Geometry: see drawing. Coordinates: mm, zero at the bounding-box minimum. A direction names the side the tool comes from. Round coordinates to 2 decimals unless told otherwise and drop trailing zeros. Order: outer loops, then holes, each group sorted by start corner. A loop starts at its lowest first (then second) coordinate and runs counter-clockwise, first axis right, second up.
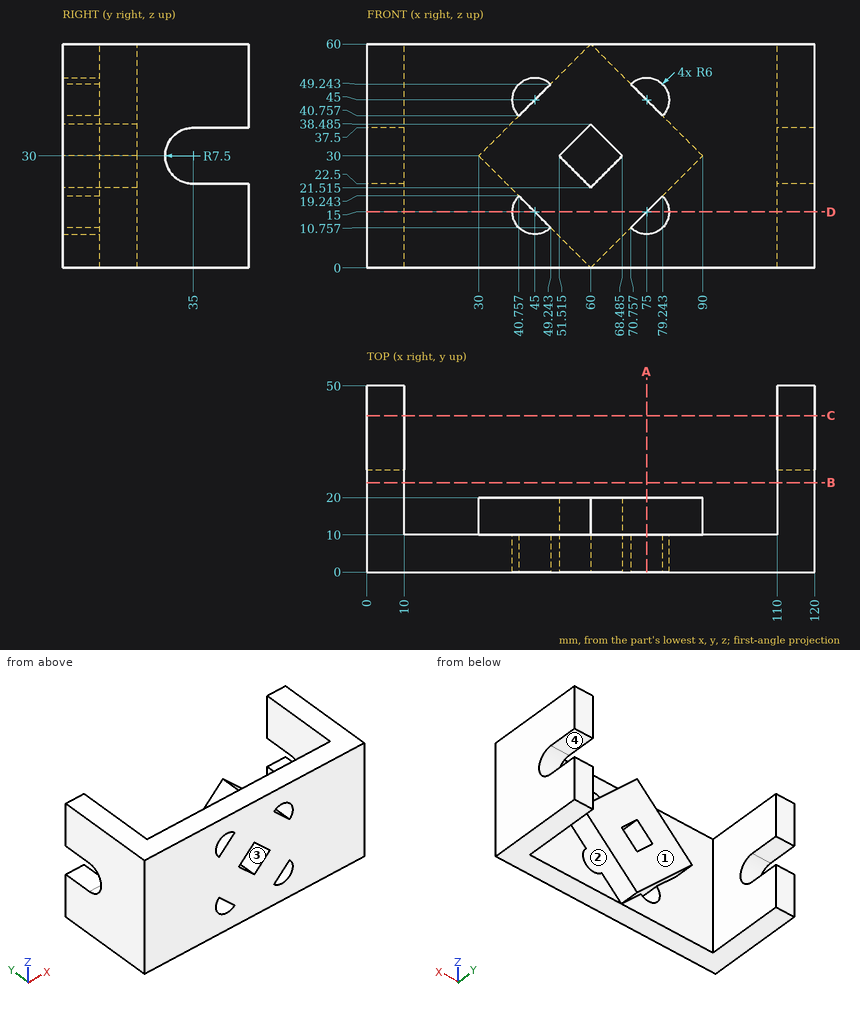
1. Line query: line 1 along X through (y, z) = (28, 51.5); line 2 along Z through (x, y) = (111, 40.5); line 3 along X through (y, z) = (13, 24) (1 decimal). Output: solid intervals per line, ascending.
2. Section C-C on y = 42. Return loops of the section in (x, z).
3. First-contact query: pin 1 (1.5 mm diameter, centred on x = 38.5, y = 19.5, fed in from +Z); pin 2 (1.5 mm diameter, centred on x = 73, z = 42, fed in from +Y); pin 3 (1.5 mm diameter, centred on y = 10, z = 38.5, fed in from -X); pin 4 (15 mm diameter, centred on x = 32, z = 45, fed in from +Y). Flat tips, straight axial feed; report the tip coordinate or a pass-through.
4. Access query for the marked faces 1, 2, 3 and 4. Directions: +Z, -Z, +X, -X, +Y, -Y. A direction counts if a zero-diameter tool reaches every point of the face in a straight line with its end or side. Return the directions, or none.
5. Section B-B on y = 24. Return loops of the section in (x, z).
6. Section A-A on x = 75. Return loops of the section in (y, z).
7. Section D-D on z = 15. Return loops of the section in (x, y).
Result:
1. line 1: x = 0 to 10, 110 to 120
1. line 2: z = 0 to 22.5, 37.5 to 60
1. line 3: x = 0 to 10, 36 to 57.5, 62.5 to 84, 110 to 120
2. outline: (0, 0) - (10, 0) - (10, 22.5) - (0, 22.5) - close; (0, 37.5) - (10, 37.5) - (10, 60) - (0, 60) - close; (110, 0) - (120, 0) - (120, 22.5) - (110, 22.5) - close; (110, 37.5) - (120, 37.5) - (120, 60) - (110, 60) - close
3. pin 1: stops at z = 39.25
3. pin 2: stops at y = 20
3. pin 3: stops at x = 0
3. pin 4: stops at y = 10
4. face 1: +Z, -Z, +Y
4. face 2: +Y
4. face 3: +Y, -Y
4. face 4: +X, -X, +Y
5. outline: (0, 0) - (10, 0) - (10, 60) - (0, 60) - close; (110, 0) - (120, 0) - (120, 60) - (110, 60) - close
6. outline: (0, 0) - (10, 0) - (10, 9) - (0, 9) - close; (0, 15) - (20, 15) - (20, 45) - (0, 45) - close; (0, 51) - (10, 51) - (10, 60) - (0, 60) - close
7. outline: (0, 0) - (39, 0) - (39, 10) - (10, 10) - (10, 50) - (0, 50) - close; (45, 0) - (75, 0) - (75, 20) - (45, 20) - close; (81, 0) - (120, 0) - (120, 50) - (110, 50) - (110, 10) - (81, 10) - close
